Could you check a few things on this model? Use its own coordinates, in mm. A direction names the side the tool comes from. Give positions to 0.01 mm unless a question says otherwise; leave off trailing zeros. Loops run counter-clockwise (first coordinate to the right, second up) from the corner with the lowest first, then second, coordinate; pieces in that order, holes last. Notation, with made-up numbers: (17, 4) -> (71, 4) arc R17 ccw to (71, 30) -> close; hole circle Ø10 at (81.5, -21). An arc over 180 degrees is marked (long way). Put each result on its own line as item: value.
Autodesk Inventor part; units mm, degrees
ref_plane "YZ Plane" through (0, 0, 0) normal (1, 0, 0) x (0, 1, 0)
ref_plane "XZ Plane" through (0, 0, 0) normal (0, 1, 0) x (-1, 0, 0)
ref_plane "XY Plane" through (0, 0, 0) normal (0, 0, 1) x (1, 0, 0)
sketch "Sketch1" plane through (0, 0, 0) normal (1, 0, 0) x (0, 1, 0)
  line L0 (0, 0) -> (20.1, 0)
  line L1 (20.1, 0) -> (20.1, 20.1)
  line L2 (20.1, 20.1) -> (0, 20.1)
  line L3 (0, 20.1) -> (0, 0)
  line L4 (-4, 24.1) -> (24.1, 24.1)
  line L5 (24.1, 24.1) -> (24.1, -4)
  line L6 (24.1, -4) -> (-4, -4)
  line L7 (-4, -4) -> (-4, 24.1)
  line L8 (12.55, 22.2) -> (7.55, 22.2)
  line L9 (7.55, 22.2) -> (7.55, 18)
  line L10 (7.55, 18) -> (12.55, 18)
  line L11 (12.55, 18) -> (12.55, 22.2)
  line L12 (12.55, 22.2) -> (7.55, 18) construction
  line L13 (7.55, 22.2) -> (12.55, 18) construction
  line L14 (12.55, 18) -> (15.35, 18)
  line L15 (15.35, 18) -> (15.35, 17)
  line L16 (15.35, 17) -> (12.55, 14.2)
  line L17 (12.55, 14.2) -> (7.55, 14.2)
  line L18 (7.55, 18) -> (4.75, 18)
  line L19 (4.75, 18) -> (4.75, 17)
  line L20 (4.75, 17) -> (7.55, 14.2)
  line L21 (2.1, 15.35) -> (3.1, 15.35)
  line L22 (3.1, 4.75) -> (5.9, 7.55)
  line L23 (2.1, 4.75) -> (3.1, 4.75)
  line L24 (-2.1, 12.55) -> (-2.1, 7.55)
  line L25 (2.1, 12.55) -> (-2.1, 12.55)
  line L26 (-2.1, 12.55) -> (2.1, 7.55) construction
  line L27 (-2.1, 7.55) -> (2.1, 12.55) construction
  line L28 (2.1, 7.55) -> (2.1, 4.75)
  line L29 (-2.1, 7.55) -> (2.1, 7.55)
  line L30 (2.1, 7.55) -> (2.1, 12.55)
  line L31 (5.9, 12.55) -> (5.9, 7.55)
  line L32 (2.1, 12.55) -> (2.1, 15.35)
  line L33 (3.1, 15.35) -> (5.9, 12.55)
  point P0 (10.05, 20.1)
  point P1 (0, 10.05)
  point P2 (10.05, 20.1)
  point P3 (0, 10.05)
  point P4 (0, 7.55)
  point P5 (0, 12.55)
  point P6 (7.55, 20.1)
  point P7 (12.55, 20.1)
  dimension "d0" = 20.1
  dimension "d1" = 20.1
  dimension "d2" = 4
  dimension "d3" = 5
  dimension "d4" = 4.2
  dimension "d5" = 2.8
  dimension "d6" = 1
  dimension "d7" = 3.8
  dimension "d8" = 2.8
  dimension "d9" = 5
  dimension "d10" = 1
  dimension "d11" = 135
  dimension "d12" = 5
  dimension "d13" = 4.2
  dimension "d14" = 2.8
  dimension "d15" = 1
  dimension "d16" = 3.8
  dimension "d17" = 2.8
  dimension "d18" = 5
  dimension "d19" = 1
  dimension "d20" = 135
  dimension "d21" = 7.55
  dimension "d22" = 2.1
  dimension "d23" = 90
  dimension "d24" = 7.55
  dimension "d25" = 2.1
  dimension "d26" = 90
extrude "Extrusion1" add sketch "Sketch1" against normal blind 80 contours L29 L24 L25 L3 | L3 L25 L30 L29 | L30 L32 L21 L33 L31 L22 L23 L28 | L11 L10 L9 L2 | L2 L9 L8 L11 | L14 L15 L16 L17 L20 L19 L18 L10 | L4 L5 L6 L7
sketch "Sketch2" plane through (0, -4, -4) normal (0, -1, 0) x (1, 0, 0)
  line L0 (0, 28.1) -> (0, 0)
  line L1 (0, 28.1) -> (-80, 28.1)
  line L2 (-80, 0) -> (-80, 28.1)
  line L3 (0, 0) -> (-80, 0)
  line L4 (-80, 0) -> (0, 28.1) construction
  line L5 (-80, 28.1) -> (0, 0) construction
  line L6 (-51, 35.25) -> (-51, -7.15) construction
  line L7 (-51, -7.15) -> (-29, -7.15) construction
  line L8 (-29, -7.15) -> (-29, 35.25) construction
  line L9 (-29, 35.25) -> (-51, 35.25) construction
  line L10 (-51, 35.25) -> (-29, -7.15) construction
  line L11 (-51, -7.15) -> (-29, 35.25) construction
  circle A0 centre (-29, 35.25) radius 1.6
  circle A1 centre (-29, -7.15) radius 1.6
  circle A2 centre (-51, 35.25) radius 1.6
  circle A3 centre (-51, -7.15) radius 1.6
  line L12 (-23, 28.1) -> (-57, 28.1)
  line L13 (-57, 40.1) -> (-23, 40.1)
  line L14 (-23, 0) -> (-57, 0)
  line L15 (-57, -12) -> (-23, -12)
  line L16 (-57, -12) -> (-60, -12)
  line L17 (-23, -12) -> (-20, -12)
  line L18 (-20, -12) -> (-20, 0)
  line L19 (-60, -12) -> (-60, 0)
  line L20 (-23, 40.1) -> (-20, 40.1)
  line L21 (-20, 40.1) -> (-20, 28.1)
  line L22 (0, 28.1) -> (-80, 28.1)
  line L23 (-57, 40.1) -> (-60, 40.1)
  line L24 (-60, 40.1) -> (-60, 28.1)
  point P0 (0, 4)
  point P1 (-40, 14.05)
  dimension "d29" = 42.4
  dimension "d31" = 22
  dimension "d32" = 3.2
  dimension "d35" = 42.4
  dimension "d38" = 22
  dimension "d41" = 34
  dimension "d42" = 12
  dimension "d44" = 12
  dimension "d46" = 34
  dimension "d59" = 3
  dimension "d60" = 3
  dimension "d61" = 3
  dimension "d62" = 3
extrude "Extrusion2" add sketch "Sketch2" against normal blind 3 contours L18 L17 L15 L16 L19 L3
sketch "Sketch3" plane through (0, 24.1, 24.1) normal (0, 1, 0) x (1, 0, 0)
  line L0 (0, 28.1) -> (0, 0)
  line L1 (0, 28.1) -> (-80, 28.1)
  line L2 (-80, 0) -> (-80, 28.1)
  line L3 (0, 0) -> (-80, 0)
  line L4 (0, 16.55) -> (0, 11.55) construction
  line L5 (0, 14.05) -> (-80, 14.05) construction
  line L6 (-80, 28.1) -> (-80, 0) construction
  circle A0 centre (-12, 14.05) radius 3
  circle A1 centre (-68, 14.05) radius 3
  line L7 (-68, 17.05) -> (-80, 17.05)
  line L8 (-68, 11.05) -> (-80, 11.05)
  line L9 (-12, 17.05) -> (0, 17.05)
  line L10 (0, 19.35) -> (0, 16.55)
  line L11 (-12, 11.05) -> (0, 11.05)
  line L12 (0, 8.75) -> (0, 11.55)
  point P0 (0, 24.1)
  point P1 (0, 11.05)
  point P2 (-80, 11.05)
  dimension "d49" = 6
  dimension "d50" = 6
  dimension "d51" = 12
  dimension "d52" = 12
  dimension "d53" = 6
  dimension "d54" = 6
extrude "Extrusion3" cut sketch "Sketch3" against normal up to surface (4 mm away) contours L0 L11 A0 L9 | L7 A1 L8 L2 | A0 | A1
ref_plane "Work Plane1" through (0, 24.1, -4) normal (0, -0.7071, -0.7071) x (-1, 0, 0)
mirror "Mirror1" about plane through (0, 24.1, -4) normal (0, -0.7071, -0.7071) of "Extrusion3"
extrude "Extrusão4" add sketch "Sketch2" against normal blind 3 contours L1 L24 L23 L13 L20 L21
fillet "Arredondamento3" radius 8 4 edges at (-60, -2.5, 36.1) (-20, -2.5, 36.1) (-20, -2.5, -16) (-60, -2.5, -16)
equation "\"d8\" = d5"
equation "\"d9\" = d3"
equation "\"d10\" = d6"
equation "\"d17\" = d14"
equation "\"d18\" = d12"
equation "\"d19\" = d15"
properties part number "cameraSlider2"
1. I'm going to push flat-ended pins straight in: pin 1 (4 mm diameter, centred on x = -48.5, y = 4, fed in from +Z); pin 2 (2.5 mm diameter, centred on x = -51, z = 31.25, fed in from -Y); pin 3 (5.5 mm diameter, centred on x = -30, y = 9.5, fed in from -Z). Where does each tip first touch, or does it pass through?
Recorded:
pin 1: stops at z = 24.1
pin 2: passes through
pin 3: stops at z = -4
2. If we section it at D-D (z = 31.25): List the corners of the cut face in (x, y) for me.
Recorded:
outline: (-59.35, -4) -> (-52.6, -4) -> (-52.6, -1) -> (-59.35, -1) -> close; (-49.4, -4) -> (-30.6, -4) -> (-30.6, -1) -> (-49.4, -1) -> close; (-27.4, -4) -> (-20.65, -4) -> (-20.65, -1) -> (-27.4, -1) -> close
3. For faces 4 (the face through (-74, 22, 13.05)), 5 (the face through (-40, -1, 30)), 6 (the face through (-74, 7.05, -2)), 7 (the face through (-39, 0, 16)), 8 (the face through (-6, 22, 7.05)), which set-ups out of +Z, -Z, +X, -X, +Y, -Y let a thin tool reach every point of the face, with its end or its side?
Recorded:
face 4: -X, +Y
face 5: +Z, +X, -X, +Y
face 6: -Z, -X
face 7: +X, -X
face 8: +X, +Y
4. Thinking about a two-plate mould opening in X: for faces 1 (the face through (-20, -3, 26)), 2 (the face through (-30, -3, 30)), 3 (the face through (-74, 22, 7.05)), which applies, pulls with the +X half, pulls with the -X half, needs draft (parallel to the pull), parting line crosses it, or undercut?
Recorded:
face 1: pulls with the +X half
face 2: undercut
face 3: needs draft
5. If we section it at C-C (x = -29): Count the separate pieces of the cut face and the enclosed holes in it, then the cut area to 3 significant figures.
Recorded:
separate pieces: 3
enclosed holes: 1
area: 524 mm^2
6. If we section it at B-B (z = 10.05): List the corners of the cut face in (x, y) for me.
Recorded:
outline: (-80, -4) -> (0, -4) -> (0, 5.9) -> (-80, 5.9) -> close; (-65, 20.1) -> (-15, 20.1) -> (-15, 24.1) -> (-65, 24.1) -> close
7. I need wall thicknesses on line 1 (Z direction, x = -72, y = 2.25); line 2 (Z direction, x = -29, y = -2.3); line 3 (Z direction, x = -5.5, y = 22.75). Which ranges of each line are inside material? Lowest first, please.
Recorded:
line 1: z = -4 to 0, 4.75 to 15.35, 20.1 to 24.1
line 2: z = -16 to -12.75, -9.55 to 29.65, 32.85 to 36.1
line 3: z = -4 to 7.05, 13.05 to 24.1
8. If we section it at A-A (y = 10.05): List the corners of the cut face in (x, z) for me, then the cut area to 3 significant figures.
Recorded:
outline: (-80, 14.2) -> (0, 14.2) -> (0, 24.1) -> (-80, 24.1) -> close; (-65, -4) -> (-15, -4) -> (-15, 0) -> (-65, 0) -> close
area: 992 mm^2
